```python
from build123d import *

# Parameters (mm, degrees)
REVOLVE1_ANGLE          = 45
CUT_EXTRUDE1_DEPTH      = 28.647117169
CUT_EXTRUDE1_DEPTH_BACK = 28.647117169
CUT_EXTRUDE4_START      = 13.576367639
CUT_EXTRUDE4_DEPTH      = 0.380999994
CUT_EXTRUDE4_START_2    = 13.957367633
CUT_EXTRUDE4_2_DEPTH    = 0.642564002
CUT_EXTRUDE5_DEPTH      = 28.732730484
CUT_EXTRUDE5_DEPTH_BACK = 28.732730484
SKETCH9_R               = 2.6035


with BuildPart() as part:
    # Sketch1 → Revolve1 (revolve, symmetric)
    with BuildSketch(Plane(origin=(0, 0, 0), x_dir=(0, 0, -1), z_dir=(1, 0, 0))) as revolve1_sk:
        with BuildLine():
            Line((-14.217802221, 0.25), (-19.048359509, 0.25))
            ThreePointArc((-19.048359509, 0.25), (-14.676690222, 12.144845166), (-3.81, 18.66511184))
            Line((-3.81, 18.66511184), (-3.81, 13.700083941))
            ThreePointArc((-3.81, 13.700083941), (-11.246181696, 8.70240181), (-14.217802221, 0.25))
        make_face()
    revolve(axis=Axis((0, 0, 0), (0, 1, 0)), revolution_arc=REVOLVE1_ANGLE / 2)
    revolve(revolve1_sk.sketch, axis=Axis((0, 0, 0), (0, -1, 0)), revolution_arc=REVOLVE1_ANGLE / 2)

    # Sketch2 → Cut-Extrude1 (cut, two sides: drawn at the far end of the back side and taken through both)
    with BuildSketch(Plane(origin=(0, 0, 0), x_dir=(1, 0, 0), z_dir=(0, 1, 0)).offset(-CUT_EXTRUDE1_DEPTH_BACK)):
        with BuildLine():
            Line((7.289491598, -17.598389479), (1.458023877, -3.519981019))
            ThreePointArc((1.458023877, -3.519981019), (1.400077392, -3.543428184), (1.341754023, -3.5659215))
            Line((1.341754023, -3.5659215), (7.173849701, -17.645845983))
            ThreePointArc((7.173849701, -17.645845983), (7.231709577, -17.622212591), (7.289491598, -17.598389479))
        make_face()
        with BuildLine():
            Line((-7.173849701, -17.645845983), (-1.341754023, -3.5659215))
            ThreePointArc((-1.341754023, -3.5659215), (-1.400077392, -3.543428184), (-1.458023877, -3.519981019))
            Line((-1.458023877, -3.519981019), (-7.289491598, -17.598389479))
            ThreePointArc((-7.289491598, -17.598389479), (-7.231709577, -17.622212591), (-7.173849701, -17.645845983))
        make_face()
    extrude(amount=CUT_EXTRUDE1_DEPTH + CUT_EXTRUDE1_DEPTH_BACK, mode=Mode.SUBTRACT)

    # Cut-Extrude4: read off the stored shape, not the designer's step
    # Cut-Extrude4 outline → Cut-Extrude4 (cut)
    with BuildSketch(Plane(origin=(0, 0, 0), x_dir=(-1, 0, 0), z_dir=(0, 0.3826834323650899, 0.9238795325112868)).offset(CUT_EXTRUDE4_START)):
        with BuildLine():
            add(Edge.make_bspline(
                [(-0.968782051, 0.862639779), (-0.953500776, 0.704297035), (-0.923044848, 0.542890698), (-0.855145508, 0.398864139), (-0.808724978, 0.30039795), (-0.745897012, 0.207923685), (-0.670245705, 0.129565817), (-0.594412641, 0.051019689), (-0.503545716, -0.015548318), (-0.405099082, -0.062878158), (-0.311601318, -0.107828748), (-0.209546118, -0.137449131), (-0.106757843, -0.151684794), (-0.05109477, -0.159393852), (0.005262189, -0.1617206), (0.061439303, -0.163129452)],
                knots=[0, 0, 0, 0, 0.29838771, 0.29838771, 0.29838771, 0.500936586, 0.500936586, 0.500936586, 0.704289141, 0.704289141, 0.704289141, 0.896734057, 0.896734057, 0.896734057, 1, 1, 1, 1], degree=3))
            Line((-0.968782051, 0.862639779), (-1.367692308, 0.862639779))
            add(Edge.make_bspline(
                [(0.081919071, -0.619026887), (-0.086162496, -0.61531723), (-0.257167265, -0.593217389), (-0.415863302, -0.537759882), (-0.576051263, -0.481781012), (-0.72706091, -0.391594396), (-0.854625463, -0.279801274), (-0.966467496, -0.181786819), (-1.065524634, -0.066561713), (-1.143726934, 0.059834888), (-1.232584949, 0.203454079), (-1.294864437, 0.365862515), (-1.329447249, 0.531081722), (-1.352245152, 0.639998589), (-1.362236386, 0.751562149), (-1.367692308, 0.862639779)],
                knots=[0, 0, 0, 0, 0.219321271, 0.219321271, 0.219321271, 0.441568871, 0.441568871, 0.441568871, 0.635043827, 0.635043827, 0.635043827, 0.85588519, 0.85588519, 0.85588519, 1, 1, 1, 1], degree=3))
            add(Edge.make_bspline(
                [(1.424679487, 0.702363337), (1.419981236, 0.545512864), (1.398709626, 0.385831481), (1.345210286, 0.238274474), (1.291294192, 0.089568013), (1.206545942, -0.050106462), (1.103378814, -0.170072469), (1.007347044, -0.281741256), (0.89204272, -0.380253902), (0.763987364, -0.453127945), (0.63762939, -0.525036038), (0.495452933, -0.572269115), (0.352111836, -0.596853545), (0.263052547, -0.612128103), (0.172266933, -0.616929095), (0.081919071, -0.619026887)],
                knots=[0, 0, 0, 0, 0.2250597, 0.2250597, 0.2250597, 0.452233869, 0.452233869, 0.452233869, 0.663328732, 0.663328732, 0.663328732, 0.871773853, 0.871773853, 0.871773853, 1, 1, 1, 1], degree=3))
            add(Edge.make_bspline(
                [(0.525350561, 2.297113938), (0.632201272, 2.182552925), (0.739042665, 2.067510357), (0.841026473, 1.948138788), (0.943081147, 1.828684271), (1.042867018, 1.706551704), (1.132291654, 1.577154573), (1.222325588, 1.446875791), (1.302241046, 1.306213708), (1.351938808, 1.155861709), (1.399991449, 1.01048674), (1.419363896, 0.85539296), (1.424679487, 0.702363337)],
                knots=[0, 0, 0, 0, 0.250309738, 0.250309738, 0.250309738, 0.500902382, 0.500902382, 0.500902382, 0.754675063, 0.754675063, 0.754675063, 1, 1, 1, 1], degree=3))
            Line((0.525350561, 2.297113938), (-0.586789864, 3.484050036))
            Line((-0.586789864, 3.484050036), (1.481666667, 3.484050036))
            Line((1.481666667, 3.484050036), (1.481666667, 3.939947472))
            Line((1.481666667, 3.939947472), (-1.538653846, 3.939947472))
            Line((-1.538653846, 3.939947472), (0.185208333, 2.100330084))
            add(Edge.make_bspline(
                [(1.025769231, 0.737980324), (1.015103197, 1.014455984), (0.898431748, 1.272392114), (0.563340129, 1.703651021), (0.374186439, 1.903082751), (0.185208333, 2.100330084)],
                knots=[0, 0, 0, 0, 0.5, 0.5, 1, 1, 1, 1], degree=3))
            add(Edge.make_bspline(
                [(0.061439303, -0.163129452), (0.181431455, -0.159946897), (0.303817751, -0.144655767), (0.416529018, -0.103477757), (0.530319754, -0.061905373), (0.636925683, 0.00439439), (0.726940524, 0.085370693), (0.806313998, 0.156774146), (0.876464564, 0.241486679), (0.926661814, 0.335660386), (0.975537276, 0.427354324), (1.007932207, 0.529885904), (1.019839954, 0.633102375), (1.023852868, 0.667886351), (1.024847174, 0.702980304), (1.025769231, 0.737980324)],
                knots=[0, 0, 0, 0, 0.246669413, 0.246669413, 0.246669413, 0.496293306, 0.496293306, 0.496293306, 0.715573497, 0.715573497, 0.715573497, 0.929171565, 0.929171565, 0.929171565, 1, 1, 1, 1], degree=3))
        make_face()
    extrude(amount=CUT_EXTRUDE4_DEPTH, mode=Mode.SUBTRACT)

    # Cut-Extrude4 2 outline → Cut-Extrude4 2 (cut)
    with BuildSketch(Plane(origin=(0, 0, 0), x_dir=(1, 0, 0), z_dir=(0, 0.38268343236508995, 0.9238795325112867)).offset(CUT_EXTRUDE4_START_2)):
        with BuildLine():
            add(Edge.make_bspline(
                [(0.968782051, -0.862639779), (0.953500776, -0.704297035), (0.923044848, -0.542890698), (0.855145508, -0.398864139), (0.808724978, -0.30039795), (0.745897012, -0.207923685), (0.670245705, -0.129565817), (0.594412641, -0.051019689), (0.503545716, 0.015548318), (0.405099082, 0.062878158), (0.311601318, 0.107828748), (0.209546118, 0.137449131), (0.106757843, 0.151684794), (0.05109477, 0.159393852), (-0.005262189, 0.1617206), (-0.061439303, 0.163129452)],
                knots=[0, 0, 0, 0, 0.29838771, 0.29838771, 0.29838771, 0.500936586, 0.500936586, 0.500936586, 0.704289141, 0.704289141, 0.704289141, 0.896734057, 0.896734057, 0.896734057, 1, 1, 1, 1], degree=3))
            Line((0.968782051, -0.862639779), (1.367692308, -0.862639779))
            add(Edge.make_bspline(
                [(-0.081919071, 0.619026887), (0.086162496, 0.61531723), (0.257167265, 0.593217389), (0.415863302, 0.537759882), (0.576051263, 0.481781012), (0.72706091, 0.391594396), (0.854625463, 0.279801274), (0.966467496, 0.181786819), (1.065524634, 0.066561713), (1.143726934, -0.059834888), (1.232584949, -0.203454079), (1.294864437, -0.365862515), (1.329447249, -0.531081722), (1.352245152, -0.639998589), (1.362236386, -0.751562149), (1.367692308, -0.862639779)],
                knots=[0, 0, 0, 0, 0.219321271, 0.219321271, 0.219321271, 0.441568871, 0.441568871, 0.441568871, 0.635043827, 0.635043827, 0.635043827, 0.85588519, 0.85588519, 0.85588519, 1, 1, 1, 1], degree=3))
            add(Edge.make_bspline(
                [(-1.424679487, -0.702363337), (-1.419981236, -0.545512864), (-1.398709626, -0.385831481), (-1.345210286, -0.238274474), (-1.291294192, -0.089568013), (-1.206545942, 0.050106462), (-1.103378814, 0.170072469), (-1.007347044, 0.281741256), (-0.89204272, 0.380253902), (-0.763987364, 0.453127945), (-0.63762939, 0.525036038), (-0.495452933, 0.572269115), (-0.352111836, 0.596853545), (-0.263052547, 0.612128103), (-0.172266933, 0.616929095), (-0.081919071, 0.619026887)],
                knots=[0, 0, 0, 0, 0.2250597, 0.2250597, 0.2250597, 0.452233869, 0.452233869, 0.452233869, 0.663328732, 0.663328732, 0.663328732, 0.871773853, 0.871773853, 0.871773853, 1, 1, 1, 1], degree=3))
            add(Edge.make_bspline(
                [(-0.525350561, -2.297113938), (-0.632201272, -2.182552925), (-0.739042665, -2.067510357), (-0.841026473, -1.948138788), (-0.943081147, -1.828684271), (-1.042867018, -1.706551704), (-1.132291654, -1.577154573), (-1.222325588, -1.446875791), (-1.302241046, -1.306213708), (-1.351938808, -1.155861709), (-1.399991449, -1.01048674), (-1.419363896, -0.85539296), (-1.424679487, -0.702363337)],
                knots=[0, 0, 0, 0, 0.250309738, 0.250309738, 0.250309738, 0.500902382, 0.500902382, 0.500902382, 0.754675063, 0.754675063, 0.754675063, 1, 1, 1, 1], degree=3))
            Line((-0.525350561, -2.297113938), (0.586789864, -3.484050036))
            Line((0.586789864, -3.484050036), (-1.481666667, -3.484050036))
            Line((-1.481666667, -3.484050036), (-1.481666667, -3.939947472))
            Line((-1.481666667, -3.939947472), (1.538653846, -3.939947472))
            Line((1.538653846, -3.939947472), (-0.185208333, -2.100330084))
            add(Edge.make_bspline(
                [(-1.025769231, -0.737980324), (-1.015103197, -1.014455984), (-0.898431748, -1.272392114), (-0.563340129, -1.703651021), (-0.374186439, -1.903082751), (-0.185208333, -2.100330084)],
                knots=[0, 0, 0, 0, 0.5, 0.5, 1, 1, 1, 1], degree=3))
            add(Edge.make_bspline(
                [(-0.061439303, 0.163129452), (-0.181431455, 0.159946897), (-0.303817751, 0.144655767), (-0.416529018, 0.103477757), (-0.530319754, 0.061905373), (-0.636925683, -0.00439439), (-0.726940524, -0.085370693), (-0.806313998, -0.156774146), (-0.876464564, -0.241486679), (-0.926661814, -0.335660386), (-0.975537276, -0.427354324), (-1.007932207, -0.529885904), (-1.019839954, -0.633102375), (-1.023852868, -0.667886351), (-1.024847174, -0.702980304), (-1.025769231, -0.737980324)],
                knots=[0, 0, 0, 0, 0.246669413, 0.246669413, 0.246669413, 0.496293306, 0.496293306, 0.496293306, 0.715573497, 0.715573497, 0.715573497, 0.929171565, 0.929171565, 0.929171565, 1, 1, 1, 1], degree=3))
        make_face()
    extrude(amount=CUT_EXTRUDE4_2_DEPTH, mode=Mode.SUBTRACT)

    # Cut-Extrude4 3 outline → Cut-Extrude4 3 (revolve)
    with BuildSketch(Plane(origin=(0, 0, 0), x_dir=(1, 0, 0), z_dir=(0, -0.9238795325112867, 0.38268343236508995))):
        with BuildLine():
            ThreePointArc((0.174307658, 14.599931635), (2.22533499, 14.425795626), (4.229733075, 13.957367633))
            Line((4.229733075, 13.957367633), (4.229733075, 14.599931635))
            Line((4.229733075, 14.599931635), (0.174307658, 14.599931635))
        make_face()
    revolve(axis=Axis((0, 0, 0), (0, 0.38268343236508995, 0.9238795325112867)))

    # Sketch9 → Cut-Extrude5 (cut, two sides: drawn at the far end of the back side and taken through both)
    with BuildSketch(Plane(origin=(8.561597025, 18.858537854, 16.803080265), x_dir=(0.9470724962077209, -0.23968096505674558, -0.2135573035893259), z_dir=(0.32101976096009477, 0.7071067811865476, 0.6300367553350547)).offset(-CUT_EXTRUDE5_DEPTH_BACK)):
        Circle(SKETCH9_R)
    extrude(amount=CUT_EXTRUDE5_DEPTH + CUT_EXTRUDE5_DEPTH_BACK, mode=Mode.SUBTRACT)


solid = part.part
```
Work out the finished part from the listing and answer in its coordinate system (mm). A direction names the side the tool comes from. Round coordinates to 2 decimals unless told otherwise and drop trailing zeros. Loops run counter-clockwise (first coordinate to the right, second up) from the corner with the lowest first, then second, coordinate; pieces in that order, holes last.
(1) The mould has two halves that part along X. Classify faces 3 (the flat face through (0, 0.25, 16)), 4 (the flat face through (2.496, 15.106, 6.351)), 5 (the flat face through (0.02, 2.73, 14.12)): pulls with the +X half, pulls with the -X half, needs draft (parallel to the pull), parting line crosses it, or undercut.
Computed values:
face 3: needs draft
face 4: pulls with the +X half
face 5: undercut
(2) The part is cut by section B-B, the plane z = 16.5. Give the vertices of the cut face in (x, y).
Computed values:
outline: (-6.7, 0.25) - (6.7, 0.25) - (6.7, 6.77) arc R9.52 ccw to (-6.7, 6.77) - close
(3) For faces 1 (the cylindrical face through (2.89, 11.72, 11.39)), 2 (the flat face through (0.689, 2.594, 14.188)), determine the directions among +Z, -Z, +X, -X, +Y, -Y from which every point of the face is accessible in a straight line to the end or side of a thin tool.
Computed values:
face 1: +X
face 2: none
(4) Find the intervals of material crossed by L1, parallel to Y at x = 0.75, z = 12.5; L2, parallel to Z at x = -6, y = 10; L3, parallel to Z at x = 5, y = 11.75, in increasing order.
Computed values:
L1: y = 6.74 to 14.36
L2: z = 14.81 to 15.06
L3: z = 13.69 to 14.14
(5) Each of these flat-tipped pins is pushed along its axis until it touches: P1, Ø3, axis at x = 0, z = 7, coming from the +Y side; P2, Ø5, axis at x = -4.5, y = 14, coming from the -Z side; P3, Ø3, axis at x = 0.5, z = 10, coming from the -Y side; P4, Ø5, axis at x = -2.5, y = 15.5, coming from the -Z side. Where does it stop, or does it pass through?
Computed values:
P1: stops at y = 18.24
P2: stops at z = 5.16
P3: stops at y = 8.35
P4: stops at z = 3.57
(6) The part is cut by section C-C, the plane x = 6.5. Give the vertices of the cut face in (y, z), and give its area (3 significant figures).
Computed values:
outline: (0.25, 16.02) - (8, 16.02) arc R17.91 ccw to (0.25, 17.91) - close
area: 9.71 mm2
(7) The part is cut by section A-A, the plane x = -3.5. Give the vertices of the cut face in (y, z), and give its area (3 significant figures).
Computed values:
outline: (0.25, 13.78) arc R13.78 cw to (10.63, 8.78) - (16.54, 8.78) arc R18.73 ccw to (0.25, 18.72) - close
area: 79.1 mm2
